Verification items for the finished model (mm, model axes). Face numbers are marked on the shaded views. Round coordinates to 2 decimals unless told otherwise and drop trailing zeros. Write each loop counter-clockwise with the first axis right and the second up, starting at its lowest first coordinate (ties: lowest second). Pieces come first, ordered by that corner, then holes. Notation, with made-up numbers: M 31,12.25 L 49,12.25 A25 ccw 49,24.25 Z; hole C 84,86 d10. An arc over 180 degrees is marked long. One line per item, written item: value. Start each with the question number.
Item 1: Section check B-B, the plane z = 35. Record the cut outline in (x, y), then the cut area to 3 significant figures.
Item 2: Gauge pin test, flat ends, axial feed: pin 1 (12 mm diameter, centred on x = -11.5, y = -16, fed in from +Z); pin 2 (4 mm diameter, centred on x = 14, z = 62.5, fed in from +Y); pin 3 (12 mm diameter, centred on y = -20.5, z = 41.5, fed in from -X); pin 4 (1.5 mm diameter, centred on x = -10.5, z = 33, fed in from +Y). Record the tip position at first contact, or that the pin passes through.
Item 3: Thickness scan on probe 1 along Y at (x, z) = (0, 57.25); probe 2 along Z at (x, y) = (-17.5, 7.5); probe 3 along Z at (x, y) = (-22, 4). Record the ranges inside material, lowest first. Write a range as from..to.
Item 4: Section check A-A, the plane z = 20.5. Record the cut outline in (x, y), then the cut area to 3 significant figures.
Item 5: Draft check along Z on the marked faces 1, 2 and 3. Enter one of: +Z half, -Z half, draft (parallel to the pull), parting line (faces both ways), or undercut.
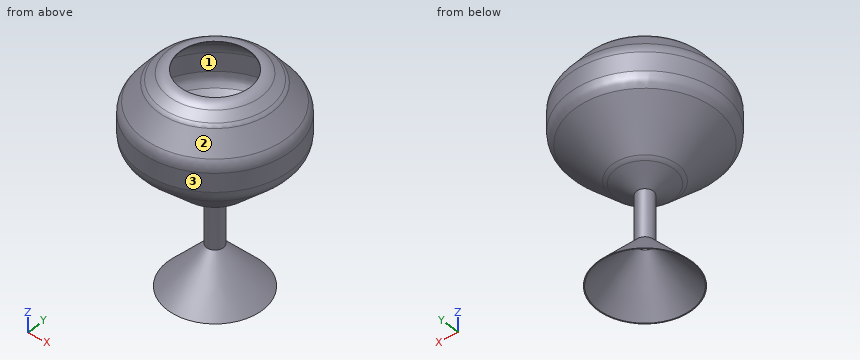
from build123d import *

# Parameters (mm, degrees)
F2_T = 0.254


# Not quite as in the source:
# - a shell that OpenCascade refuses in one call is made with other operations: the cavity is built on its own and cut out
# - a feature names something its author has since deleted; it is built from what else it names


with BuildPart() as f1:
    # F0 (on Front) → F1 (revolve)
    with BuildSketch(Plane.XZ):
        with BuildLine():
            Line((-3.0112911481, 31.8550616503), (-3.0112911481, 14.9488672614))
            Line((-3.0112911481, 14.9488672614), (-17.0688, 0))
            Line((-17.0688, 0), (0, 0))
            Line((0, 0), (0, 76.0556012392))
            Line((0, 76.0556012392), (-12.6169178095, 76.228944836))
            ThreePointArc((-12.6169178095, 76.228944836), (-14.7075461422, 75.9052317699), (-16.5758116747, 74.9127092893))
            Line((-16.5758116747, 74.9127092893), (-19.5062669903, 72.6585163811))
            ThreePointArc((-19.5062669903, 72.6585163811), (-20.0880647436, 72.1518528829), (-20.6041254437, 71.57837413))
            Line((-20.6041254437, 71.57837413), (-25.8698135255, 64.9586474103))
            ThreePointArc((-25.8698135255, 64.9586474103), (-26.8952491924, 63.0991932265), (-27.2502955049, 61.005624435))
            Line((-27.2502955049, 61.005624435), (-27.2502955049, 54.34028509))
            ThreePointArc((-27.2502955049, 54.34028509), (-26.7348850464, 51.8342793274), (-25.2723223137, 49.735083511))
            Line((-25.2723223137, 49.735083511), (-11.7529370155, 36.9002240705))
            ThreePointArc((-11.7529370155, 36.9002240705), (-11.1278091674, 36.3787066033), (-10.4410949941, 35.9414550289))
            Line((-10.4410949941, 35.9414550289), (-3.0112911481, 31.8550616503))
        make_face()
    revolve(axis=Axis((0, 0, 38.0278006196), (0, 0, -1)))

    # F2: shell of thickness 0.254, made by hand


with BuildPart() as f2_core1:
    # F2_t2: copy of F1
    add(f1.part)

    # the walls: a layer under each face that stays
    f2_faces = [f2_core1.faces().sort_by_distance(p)[0] for p in [
        (3.0112911481, 0, 23.4019644558),
        (10.0400455741, 0, 7.4744336307),
        (14.7075461422, 0, 75.9052317699),
        (18.0410393325, 0, 73.7856128352),
        (20.0880647436, 0, 72.1518528829),
        (23.2369694846, 0, 68.2685107702),
        (26.8952491924, 0, 63.0991932265),
        (27.2502955049, 0, 57.6729547625),
        (26.7348850464, 0, 51.8342793274),
        (18.5126296646, 0, 43.3176537907),
        (11.1278091674, 0, 36.3787066033),
        (6.7261930711, 0, 33.8982583396),
    ]]
    thicken(f2_faces, amount=-F2_T, mode=Mode.SUBTRACT)

    # F2_s3 → F2_t4 (revolve, cut)
    with BuildSketch(Plane.XZ):
        Polygon((-3.0150552221, 31.852836062), (-2.7572911481, 31.8550616503), (-2.7572911481, 32.005244518), (-2.8888837566, 32.0776204751), align=None)
    revolve(axis=Axis((0, 0, 31.8550616503), (0, 0, -1)), mode=Mode.SUBTRACT)

    # F2_s5 → F2_t6 (revolve, cut)
    with BuildSketch(Plane.XZ):
        Polygon((-3.0156815181, 14.9506072991), (-2.7572911481, 14.9488672614), (-2.7572911481, 14.8481993064), (-2.8262541531, 14.7748634958), align=None)
    revolve(axis=Axis((0, 0, 14.9488672614), (0, 0, -1)), mode=Mode.SUBTRACT)


with BuildPart() as f1_1:
    add(f1.part)

    # what is left inside the walls is the cavity
    f2_cavity = [f2_core1.part.solids().sort_by_distance(p)[0] for p in [
        (20.589231, 0, 45.642847),
    ]]
    add(f2_cavity, mode=Mode.SUBTRACT)


solid = f1_1.part
Response values:
1. outline: C 0,0 d17.46; hole C 0,0 d16.4
1. area: 28.0 mm2
2. pin 1: stops at z = 76.15
2. pin 2: stops at y = 24.35
2. pin 3: stops at x = -13.54
2. pin 4: passes through
3. probe 1: y = -27.25..-27, 27..27.25
3. probe 2: z = 43.82..44.17, 72.7..73.02
3. probe 3: z = 46.97..47.32, 68.96..69.37
4. outline: C 0,0 d6.02; hole C 0,0 d5.51
4. area: 4.60 mm2
5. face 1: undercut
5. face 2: +Z half
5. face 3: draft
